```python
from build123d import *

# Parameters (mm, degrees)
SKETCH_1_W      = 12.5
SKETCH_1_H      = 31.8
SKETCH_1_R      = 1
EXTRUDE_1_DEPTH = 3
SKETCH_2_W      = 12.5
SKETCH_2_H      = 22.4
EXTRUDE_2_DEPTH = 11
SKETCH_3_W      = 12.5
SKETCH_3_H      = 22.4
EXTRUDE_4_DEPTH = 16


with BuildPart() as part:
    # 草图1 → 凸台-拉伸1 (new body)
    with BuildSketch(Plane.XY):
        with Locations((0, -14)):
            Rectangle(SKETCH_1_W, SKETCH_1_H)
        Circle(SKETCH_1_R, mode=Mode.SUBTRACT)
        with Locations((0, -28)):
            Circle(SKETCH_1_R, mode=Mode.SUBTRACT)
    extrude(amount=EXTRUDE_1_DEPTH)

    # 草图2 → 凸台-拉伸2 (add)
    with BuildSketch(Plane.XY.offset(3)):
        with Locations((0, -14)):
            Rectangle(SKETCH_2_W, SKETCH_2_H)
    extrude(amount=EXTRUDE_2_DEPTH)

    # 草图3 → 凸台-拉伸4 (add)
    with BuildSketch(Plane(origin=(0, 0, 0), x_dir=(-1, 0, 0), z_dir=(0, 0, -1))):
        with Locations((0, -14)):
            Rectangle(SKETCH_3_W, SKETCH_3_H)
    extrude(amount=EXTRUDE_4_DEPTH)


solid = part.part
```
Design review of the part built by this model. Coordinates are the model's own, in mm. A direction names the side the tool comes from. Give positions to 0.01 mm unless a question says otherwise; leave off trailing zeros. Order: outer loops, then holes, each group sorted by start corner. A loop starts at its lowest first (then second) coordinate and runs counter-clockwise, first axis right, second up. Notation, with made-up numbers: (11.5, 15) -> (50.5, 15) arc R12 cw to (50.5, 33) -> close; hole circle Ø9 at (17, 39.25). An arc over 180 degrees is marked (long way). Write each question's results on one line, items separated by ' | '. Start each with the question number.
Q1. Machinability: for faces 1 (the flat face through (0, -25.2, -8)), 2 (the flat face through (0, -2.8, 8)), 3 (the flat face through (0, -26, 3)), 4 (the flat face through (0, -2.8, -8)), 5 (the flat face through (0, -14, 14)), which of the approach directions +Z, -Z, +X, -X, +Y, -Y give a long, thin tool a straight path to every point of the face, cutting with its end or side? Answer none if there is none.
Q2. Wall thickness on L1, parallel to Y at x = 0, z = 1.5; L2, parallel to Y at x = -5.25, z = -6.75; L3, parallel to Z at x = -3, y = -2.5: over which ranges is each line inside the solid? List them lowest first. Write a range as from..to.
Q3. Add section D-D on z = -2.5. Give the boundary of the cut face in (x, y).
Q4. Mouldability with a two-part tool opening along X and no side actions: class faces 6 (the flat face through (6.25, -14, -1)), 7 (the cylindrical face through (0, -27, 1)), 8 (the flat face through (0, -29.9, 1)), 9 (the flat face through (-6.25, -14, -1)) as +X half, -X half, draft (parallel to the pull), parting line (faces both ways), or undercut.
Q5. Add section B-B on x = 0. Give the boundary of the cut face in (y, z).
Q6. Add section C-C on x = 4.75. Give the boundary of the cut face in (y, z).
Q7. Add section A-A on y = 0. Give the boundary of the cut face in (x, z).
Q8. For pin 1 (5 mm diameter, centred on x = -0.5, y = 0, fed in from +Z); pin 2 (2.5 mm diameter, centred on x = 1, y = 0.5, fed in from -Z); pin 3 (1 mm diameter, centred on x = 2.5, z = -3, fed in from -Y); pin 4 (1.2 mm diameter, centred on x = 0, y = -28, fed in from -Z), all flat-tipped, find the tip position at first contact; note any pin that passes through.
Found:
1) face 1: -Z, +X, -X, -Y | face 2: +Z, +X, -X, +Y | face 3: +Z, +X, -X, -Y | face 4: -Z, +X, -X, +Y | face 5: +Z, +X, -X, +Y, -Y
2) L1: y = -29.9..-29, -27..-1, 1..1.9 | L2: y = -25.2..-2.8 | L3: z = 0..3
3) outline: (-6.25, -25.2) -> (6.25, -25.2) -> (6.25, -2.8) -> (-6.25, -2.8) -> close
4) face 6: +X half | face 7: undercut | face 8: draft | face 9: -X half
5) outline: (-29.9, 0) -> (-29, 0) -> (-29, 3) -> (-29.9, 3) -> close; (-27, 0) -> (-25.2, 0) -> (-25.2, -16) -> (-2.8, -16) -> (-2.8, 0) -> (-1, 0) -> (-1, 3) -> (-2.8, 3) -> (-2.8, 14) -> (-25.2, 14) -> (-25.2, 3) -> (-27, 3) -> close; (1, 0) -> (1.9, 0) -> (1.9, 3) -> (1, 3) -> close
6) outline: (-29.9, 0) -> (-25.2, 0) -> (-25.2, -16) -> (-2.8, -16) -> (-2.8, 0) -> (1.9, 0) -> (1.9, 3) -> (-2.8, 3) -> (-2.8, 14) -> (-25.2, 14) -> (-25.2, 3) -> (-29.9, 3) -> close
7) outline: (-6.25, 0) -> (-1, 0) -> (-1, 3) -> (-6.25, 3) -> close; (1, 0) -> (6.25, 0) -> (6.25, 3) -> (1, 3) -> close
8) pin 1: stops at z = 3 | pin 2: stops at z = 0 | pin 3: stops at y = -25.2 | pin 4: passes through
